Build history of the part. All positions in model axes, mm. Give positions to 0.01 mm unless a question says otherwise; leave off trailing zeros. Write each loop counter-clockwise with the first axis right and the second up, starting at its lowest first coordinate (ties: lowest second). Pieces come first, ordered by that corner, then holes. Notation, with made-up numbers: M -27.5,49.25 L -11.5,49.25 A14 ccw -11.5,69.25 Z; hole C -11.75,83 d8. An arc over 180 degrees is marked long. Return JSON: item names as keys, results as strings. Group by question number.
Q1. Band-saw the part on C-C, the plane x = 48.5. Give the cut face in (y, z), then the cut area to 3 significant figures.
Q2. Flat gauge pins, fed straight in: pin 1 Ø11 at (x, y) = (-505, -95) entering from -Z; pin 2 Ø1 at (x, y) = (-148, 3.5) entering from +Z; pin 3 Ø22.5 at (x, y) = (-489.5, -84.5) entering from +Z; pin 4 Ø5 at (x, z) = (201.5, 9.5) entering from -Y. Where does each tip first touch, or does it go through?
Q3. Band-saw the part on B-B, the plane y = 0. Give the cut face in (x, z), then the cut area to 3 significant figures.
Q4. Band-saw the part on A-A, the plane z = 30. Give the cut face in (x, y).
Q5. Band-saw the part on D-D, the plane y = -66. Give the cut face in (x, z).
Q6. Wall check: probe 1 along Y at (x, z) = (-505, 6); probe 2 along Y at (x, z) = (505, 11.25); probe 3 along Y at (x, z) = (-76.5, 20.5). Give the ranges that are in metal, low to high.
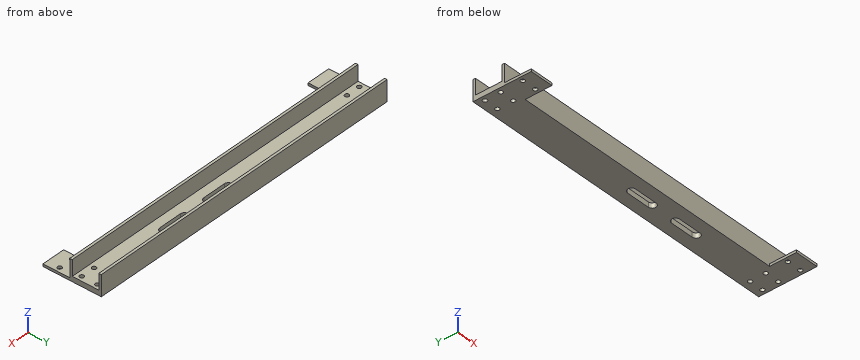
from build123d import *

# Parameters (mm, degrees)
BOSS_EXTRUDE1_DEPTH     = 8
SKETCH2_W               = 1040
SKETCH2_H               = 100
BOSS_EXTRUDE2_DEPTH     = 8
CUT_EXTRUDE1_DEPTH      = 538.476511115
CUT_EXTRUDE1_DEPTH_BACK = 538.476511115
SKETCH4_W               = 1040
SKETCH4_H               = 8
BOSS_EXTRUDE3_DEPTH     = 50
F_12_0MM_DOWEL_HOLE1_D  = 13.5


with BuildPart() as part:
    # Sketch1 → Boss-Extrude1 (new body)
    with BuildSketch(Plane.XY):
        Polygon((-445, -50), (445, -50), (445, -135), (520, -135), (520, -50), (520, 50), (-520, 50), (-520, -50), (-520, -135), (-445, -135), align=None)
    extrude(amount=BOSS_EXTRUDE1_DEPTH)

    # Sketch2 → Boss-Extrude2 (add)
    with BuildSketch(Plane.XY.offset(8)):
        Rectangle(SKETCH2_W, SKETCH2_H)
    extrude(amount=BOSS_EXTRUDE2_DEPTH)

    # Sketch3 → Cut-Extrude1 (cut, two sides: drawn at the far end of the back side and taken through both)
    with BuildSketch(Plane.XY.offset(16).offset(-CUT_EXTRUDE1_DEPTH_BACK)):
        with BuildLine():
            Line((0, 12.5), (75, 12.5))
            ThreePointArc((75, 12.5), (87.5, 0), (75, -12.5))
            Line((75, -12.5), (0, -12.5))
            ThreePointArc((0, -12.5), (-12.5, 0), (0, 12.5))
        make_face()
        with BuildLine():
            Line((160, 12.5), (235, 12.5))
            ThreePointArc((235, 12.5), (247.5, 0), (235, -12.5))
            Line((235, -12.5), (160, -12.5))
            ThreePointArc((160, -12.5), (147.5, 0), (160, 12.5))
        make_face()
    extrude(amount=CUT_EXTRUDE1_DEPTH + CUT_EXTRUDE1_DEPTH_BACK, mode=Mode.SUBTRACT)

    # Sketch4 → Boss-Extrude3 (add)
    with BuildSketch(Plane.XY.offset(16)):
        with Locations((0, 46)):
            Rectangle(SKETCH4_W, SKETCH4_H)
        with Locations((0, -46)):
            Rectangle(SKETCH4_W, SKETCH4_H)
    extrude(amount=BOSS_EXTRUDE3_DEPTH)

    # Ø12.0mm Dowel Hole1 (through all)
    with Locations(Plane.XY.offset(16)):
        with Locations((-460, 25), (-505, 25), (-505, -25), (-460, -25), (-460, -95), (-505, -95), (460, -95), (505, -95), (505, -25), (460, -25), (460, 25), (505, 25)):
            Hole(F_12_0MM_DOWEL_HOLE1_D / 2)


solid = part.part
From the geometry:
{
 "1": {"outline": "M -50,0 L -12.5,0 L -12.5,16 L -42,16 L -42,66 L -50,66 Z; M 12.5,0 L 50,0 L 50,66 L 42,66 L 42,16 L 12.5,16 Z", "area": "2,000 mm^2"},
 "2": {"pin 1": "passes through", "pin 2": "stops at z = 16", "pin 3": "stops at z = 8", "pin 4": "stops at y = -50"},
 "3": {"outline": "M -520,0 L -12.5,0 L -12.5,16 L -520,16 Z; M 87.5,0 L 147.5,0 L 147.5,16 L 87.5,16 Z; M 247.5,0 L 520,0 L 520,16 L 247.5,16 Z", "area": "13,400 mm^2"},
 "4": {"outline": "M -520,-50 L 520,-50 L 520,-42 L -520,-42 Z; M -520,42 L 520,42 L 520,50 L -520,50 Z"},
 "5": {"outline": "M -520,0 L -445,0 L -445,8 L -520,8 Z; M 445,0 L 520,0 L 520,8 L 445,8 Z"},
 "6": {"probe 1": "y = -135 to -101.75, -88.25 to -31.75, -18.25 to 18.25, 31.75 to 50", "probe 2": "y = -50 to -31.75, -18.25 to 18.25, 31.75 to 50", "probe 3": "y = -50 to -42, 42 to 50"}
}
